```python
from build123d import *

# Parameters (mm, degrees)
SKETCH_W        = 69
SKETCH_H        = 43
PAD_DEPTH       = 23
THICKNESS_T     = 1.5
SKETCH001_R     = 1.5
HOLE_DEPTH      = 2.098709
HOLE_TIPS_R     = 1.5
POCKET_DEPTH    = 5
SKETCH003_W     = 8
SKETCH003_H     = 8
PAD001_DEPTH    = 3
SKETCH004_R     = 2
HOLE001_DEPTH   = 6
POCKET001_DEPTH = 3


with BuildPart() as part:
    # Sketch → Pad (new body)
    with BuildSketch(Plane.XY):
        Rectangle(SKETCH_W, SKETCH_H)
    extrude(amount=PAD_DEPTH)

    # Thickness
    thickness_openings = [part.faces().sort_by_distance(p)[0] for p in [
        (0, 0, 23),
    ]]
    offset(amount=THICKNESS_T, openings=thickness_openings)

    # Sketch001 (on Face10 of Thickness) → Hole (cut)
    with BuildSketch(Plane.YZ.offset(36)):
        with Locations((0, 9)):
            Circle(SKETCH001_R)
    extrude(amount=-HOLE_DEPTH, mode=Mode.SUBTRACT)

    # Hole tips → Hole tip 1 section 0
    with BuildSketch(Plane.YZ.offset(33.901291), mode=Mode.PRIVATE) as hole_tip_1_s0:
        with Locations((0, 9)):
            Circle(HOLE_TIPS_R)
    loft([hole_tip_1_s0.sketch, Vertex(33, 0, 9)], mode=Mode.SUBTRACT)

    # Sketch002 (on Face9 of Hole) → Pocket (cut)
    with BuildSketch(Plane(origin=(-36, 0, 0), x_dir=(0, -1, 0), z_dir=(-1, 0, 0))):
        with BuildLine():
            ThreePointArc((-3, 15), (-6, 12), (-3, 9))
            Line((-3, 9), (3, 9))
            ThreePointArc((3, 9), (6, 12), (3, 15))
            Line((-3, 15), (3, 15))
        make_face()
    extrude(amount=-POCKET_DEPTH, mode=Mode.SUBTRACT)

    # Sketch003 (on Face4 of Pocket) → Pad001 (join)
    with BuildSketch(Plane.XY):
        with Locations((-28.95, 15.6)):
            Rectangle(SKETCH003_W, SKETCH003_H)
        with Locations((28.95, 15.6)):
            Rectangle(SKETCH003_W, SKETCH003_H)
        with Locations((-28.95, -16.25)):
            Rectangle(SKETCH003_W, SKETCH003_H)
        with Locations((28.95, -16.25)):
            Rectangle(SKETCH003_W, SKETCH003_H)
    extrude(amount=PAD001_DEPTH)

    # Sketch004 (on Face38 of Pad001) → Hole001 (cut)
    with BuildSketch(Plane.XY.offset(3)):
        with Locations((-28.95, 15.925)):
            Circle(SKETCH004_R)
        with Locations((28.95, 15.92)):
            Circle(SKETCH004_R)
        with Locations((-28.95, -15.925)):
            Circle(SKETCH004_R)
        with Locations((28.95, -15.93)):
            Circle(SKETCH004_R)
    extrude(amount=-HOLE001_DEPTH, mode=Mode.SUBTRACT)

    # Sketch005 (on Face52 of Hole001) → Pocket001 (cut)
    with BuildSketch(Plane(origin=(0, 0, -1.5), x_dir=(1, 0, 0), z_dir=(0, 0, -1))):
        Polygon((-27.206792, 12.885), (-25.450009, 15.912163), (-27.193217, 18.947163), (-30.693208, 18.955), (-32.449991, 15.927837), (-30.706783, 12.892837), align=None)
        Polygon((30.693208, 12.89), (32.449991, 15.917163), (30.706783, 18.952163), (27.206792, 18.96), (25.450009, 15.932837), (27.193217, 12.897837), align=None)
        Polygon((-27.206792, -18.965), (-25.450009, -15.937837), (-27.193217, -12.902837), (-30.693208, -12.895), (-32.449991, -15.922163), (-30.706783, -18.957163), align=None)
        Polygon((30.693208, -18.96), (32.449991, -15.932837), (30.706783, -12.897837), (27.206792, -12.89), (25.450009, -15.917163), (27.193217, -18.952163), align=None)
    extrude(amount=-POCKET001_DEPTH, mode=Mode.SUBTRACT)


solid = part.part
```
Design review of the part built by this model. Coordinates are the model's own, in mm. A direction names the side the tool comes from. Coordinates: 2 decimals unless noted, no trailing zeros. Loops run counter-clockwise (first coordinate to the right, second up) from the corner with the lowest first, then second, coordinate; pieces in that order, holes last.
Q1. We need section A-A on z = 21.5. State the section outline as (x, y) points, and give its area (3 significant figures).
Reported:
outline: (-36, -21.5) arc R1.5 ccw to (-34.5, -23) - (34.5, -23) arc R1.5 ccw to (36, -21.5) - (36, 21.5) arc R1.5 ccw to (34.5, 23) - (-34.5, 23) arc R1.5 ccw to (-36, 21.5) - close; hole (-34.5, -21.5) - (34.5, -21.5) - (34.5, 21.5) - (-34.5, 21.5) - close
area: 343 mm2
Q2. To check wall thickness, follow line 1 (Y direction, x = -28.95, z = 2.25) (3 decimals); line 2 (X direction, y = 7.5, z = 15.5); line 3 (Y direction, x = -4, z = 5.75). State the ranges of each line that lie inside material, in increasing order.
Reported:
line 1: y = -23 to -21.5, -20.25 to -17.925, -13.925 to -12.25, 11.6 to 13.925, 17.925 to 19.6, 21.5 to 23
line 2: x = -36 to -34.5, 34.5 to 36
line 3: y = -23 to -21.5, 21.5 to 23
Q3. The part is to be moulded in two halves that separate along Y. For faces 1 (the face through (36, 0, 11)), 2 (the face through (31.56, 17.47, -0.02)), 3 (the face through (35.57, 22.55, 11.66)), say which applies: +Y half, -Y half, draft (parallel to the pull), parting line (faces both ways), or undercut.
Reported:
face 1: draft
face 2: undercut
face 3: +Y half
Q4. We need section D-D on z = 12. State the section outline as (x, y) points, and give its area (3 significant figures).
Reported:
outline: (-36, -21.5) arc R1.5 ccw to (-34.5, -23) - (34.5, -23) arc R1.5 ccw to (36, -21.5) - (36, 21.5) arc R1.5 ccw to (34.5, 23) - (-34.5, 23) arc R1.5 ccw to (-36, 21.5) - (-36, 6) - (-34.5, 6) - (-34.5, 21.5) - (34.5, 21.5) - (34.5, -21.5) - (-34.5, -21.5) - (-34.5, -6) - (-36, -6) - close
area: 325 mm2
Q5. We need section C-C on y = -10. State the section outline as (x, z) points.
Reported:
outline: (-36, 0) arc R1.5 ccw to (-34.5, -1.5) - (34.5, -1.5) arc R1.5 ccw to (36, 0) - (36, 23) - (34.5, 23) - (34.5, 0) - (-34.5, 0) - (-34.5, 23) - (-36, 23) - close
Q6. For pin 1 (0.8 mm diameter, centred on x = -35, y = 0.5, fed in from -Z); pin 2 (3.5 mm diameter, centred on x = 28.95, y = 15.92, fed in from -Z), all flat-tipped, find the tip position at first contact; note any pin that passes through.
Reported:
pin 1: stops at z = -1.5
pin 2: passes through
Q7. Tool access review of faces 4 (the face through (30.797, 15.154, 2.26)), 5 (the face through (-26.31, -17.41, -0.02)), 6 (the face through (-32.95, 16, 1)): name each direction out of +Z, -Z, +X, -X, +Y, -Y from which nothing blocks a thin tool from reaching the whole face with its end or side.
Reported:
face 4: +Z, -Z
face 5: -Z
face 6: +Z
Q8. We need section B-B on y = 0. State the section outline as (x, z) points.
Reported:
outline: (-36, 0) arc R1.5 ccw to (-34.5, -1.5) - (34.5, -1.5) arc R1.5 ccw to (36, 0) - (36, 7.5) - (34.5, 7.5) - (34.5, 0) - (-34.5, 0) - (-34.5, 9) - (-36, 9) - close; (-36, 15) - (-34.5, 15) - (-34.5, 23) - (-36, 23) - close; (34.5, 10.5) - (36, 10.5) - (36, 23) - (34.5, 23) - close
